```python
from build123d import *

# Parameters (mm, degrees)
ESQUISSE1_R                  = 10
BOSS_EXTRU_1_DEPTH           = 120
ENL_V_MAT_EXTRU_1_DEPTH      = 16
ENL_V_MAT_EXTRU_2_DEPTH      = 122.610032481
ENL_V_MAT_EXTRU_2_DEPTH_BACK = 122.610032481
ESQUISSE3_R                  = 6


with BuildPart() as part:
    # Esquisse1 → Boss.-Extru.1 (new body)
    with BuildSketch(Plane.XY):
        Circle(ESQUISSE1_R)
    extrude(amount=BOSS_EXTRU_1_DEPTH)

    # Esquisse2 → Enlèv. mat.-Extru.1 (cut)
    with BuildSketch(Plane(origin=(0, 0, 0), x_dir=(-1, 0, 0), z_dir=(0, 0, -1))):
        with BuildLine():
            Line((-7, 7.141428429), (-7, -7.141428429))
            ThreePointArc((-7, -7.141428429), (-10, 0), (-7, 7.141428429))
        make_face()
        with BuildLine():
            Line((7, 7.141428429), (7, -7.141428429))
            ThreePointArc((7, -7.141428429), (10, 0), (7, 7.141428429))
        make_face()
    extrude(amount=-ENL_V_MAT_EXTRU_1_DEPTH, mode=Mode.SUBTRACT)

    # Esquisse3 → Enlèv. mat.-Extru.2 (cut, two sides: drawn at the far end of the back side and taken through both)
    with BuildSketch(Plane(origin=(7, 0, 0), x_dir=(0, 0, -1), z_dir=(1, 0, 0)).offset(-ENL_V_MAT_EXTRU_2_DEPTH_BACK)):
        with Locations(Location((-8, 0, 0), (0, 0, 90))):
            Circle(ESQUISSE3_R)
    extrude(amount=ENL_V_MAT_EXTRU_2_DEPTH + ENL_V_MAT_EXTRU_2_DEPTH_BACK, mode=Mode.SUBTRACT)


solid = part.part
```
Here's how the part is built. I have some questions about the finished solid (model axes, mm). A direction names the side the tool comes from. Give positions to 0.01 mm unless a question says otherwise; leave off trailing zeros. Write each loop counter-clockwise with the first axis right and the second up, starting at its lowest first coordinate (ties: lowest second). Pieces come first, ordered by that corner, then holes. Notation, with made-up numbers: (78, 35.5) -> (126, 35.5) arc R26 ccw to (126, 54.5) -> close; hole circle Ø11 at (3.25, -33). An arc over 180 degrees is marked (long way). Use one line per item in the form item = value.
1) Suppose I cut it at B-B (z = 8). Please give me the cut outline in (x, y).
Verdict:
outline = (-7, -7.14) arc R10 ccw to (7, -7.14) -> (7, -6) -> (-7, -6) -> close; (-7, 6) -> (7, 6) -> (7, 7.14) arc R10 ccw to (-7, 7.14) -> close
2) Suppose I cut it at C-C (y = 0). Please give me the cut outline in (x, z).
Verdict:
outline = (-10, 16) -> (-7, 16) -> (-7, 14) -> (7, 14) -> (7, 16) -> (10, 16) -> (10, 120) -> (-10, 120) -> close; (-7, 0) -> (7, 0) -> (7, 2) -> (-7, 2) -> close
3) If I drill on L1, parallel to Z at x = -4.5, y = 0.5; L2, parallel to Y at x = 7, z = 87; L3, parallel to Y at x = -2.5, z = 8, over which ranges is the centre line in solid material (lowest first)? Write a range as [from, to].
Verdict:
L1 = [0, 2.02], [13.98, 120]
L2 = [-7.14, 7.14]
L3 = [-9.68, -6], [6, 9.68]
4) Suppose I cut it at A-A (x = 0). Please give me the cut outline in (y, z).
Verdict:
outline = (-10, 0) -> (10, 0) -> (10, 120) -> (-10, 120) -> close; hole circle Ø12 at (0, 8)
5) On a 3-axis mill with a long thin cutter (end or side, diameter ignored), from which of +Z, -Z, +X, -X, +Y, -Y can I reach the whole of each face in a straight line? I mean faces 4 (the face through (0, 0, 120)), 5 (the face through (7, 5, 4)), 6 (the face through (-7, 5, 4)). Say none if no direction works.
Verdict:
face_4 = +Z, +X, -X, +Y, -Y
face_5 = -Z, +X, +Y, -Y
face_6 = -Z, -X, +Y, -Y
6) Suppose I cut it at D-D (z = 93.5). Please give me the cut outline in (x, y).
Verdict:
outline = circle Ø20 at (0, 0)
7) I'm going to push flat-ended pins straight in: pin 1 (1.5 mm diameter, centred on x = 7.5, z = 57, fed in from -Y); pin 2 (1.5 mm diameter, centred on x = 3, z = 30, fed in from +Y); pin 3 (6 mm diameter, centred on x = -7, z = 91.5, fed in from +Y). Where does each tip first touch, or does it pass through?
Verdict:
pin_1 = -7.38
pin_2 = 9.74
pin_3 = 9.17
8) We'd pull the mould along Y, two halves only. Please class faces 1 (the face through (9.54, 3, 59.16)), 2 (the face through (8, 0, 16)), 3 (the face through (-0.098, 2.769, 2.677)): +Y half, -Y half, draft (parallel to the pull), parting line (faces both ways), or undercut.
Verdict:
face_1 = parting line
face_2 = draft
face_3 = undercut
